Check sheet for the modelled part. Datum: model origin and axes. Units: mm. A direction names the side the tool comes from. Give positions to 0.01 mm unless a question says otherwise; leave off trailing zeros. Write each loop counter-clockwise with the first axis right and the second up, starting at its lowest first coordinate (ties: lowest second). Pieces come first, ordered by that corner, then holes. Notation, with made-up numbers: (75.5, 41.25) -> (112.5, 41.25) arc R20 ccw to (112.5, 77.25) -> close; hole circle Ø11 at (5, 80.25). An arc over 180 degrees is marked (long way). Use a Markdown table: item, result. Add a question column.
1. Gauge pin test, flat ends, axial feed: P1, Ø17.5, axis at x = -26.86, z = 15.88, coming from the -Y side; P2, Ø10, axis at x = -23, z = 25, coming from the +Y side; P3, Ø13.5, axis at y = -17.5, z = 11, coming from the -X side. Record the tip position at first contact, or that the pin passes through.
2. Scan lines: probe 1 along Y at (x, z) = (-24, 23); probe 2 along Y at (x, z) = (43.5, 29); probe 3 along X at (y, z) = (-3, 13). Record each from-to range of solid material in increasing order. Write a range as [from, to].
3. Cross-section at D-D (y = 13). Enter the section's corners in (x, z), then the cut area to 3 significant figures.
4. Cross-section at C-C (x = -23.5). Enter the section's corners in (y, z).
5. Set-up check for faces 1 (the flat face through (-22, 4.854, 19)), 2 (the flat face through (-22, -5.941, 19)), 3 (the flat face through (28, 0, 16)): record each of +Z, -Z, +X, -X, +Y, -Y from which the full face is reachable in a straight line by a thin tool's end or side.
6. Release check for a two-part mould opening along X. For faces 4 (the flat face through (-7, -23.086, 16)), 5 (the flat face through (0, 29, 16)), 6 (the cylindrical face through (-21.466, -0.619, 15.638)), 7 (the flat face through (-38.161, -1, 16)) record: released by +X, released by -X, zero draft, split by the parting line, or undercut.
7. Cross-section at A-A (z = 23). Enter the section's corners in (x, y) (3 decimals).
from build123d import *
from OCP.BRepFilletAPI import BRepFilletAPI_MakeChamfer

# Parameters (mm, degrees)
BOSS_EXTRUDE1_DEPTH          = 31.75
F_3_8_0_375_DIAMETER_HOLE1_D = 10.795
FILLET1_R                    = 1.27
FILLET2_R                    = 6.35
CHAMFER1_SIZE                = 0.254
CHAMFER1_SIZE2               = 0.321383695


with BuildPart() as part:
    # Sketch1 → Boss-Extrude1 (new body)
    with BuildSketch(Plane.XY):
        Polygon((0, 0), (50.8, 0), (50.8, -9.525), (-3.3628076, -23.086314), (-11.6178076, -23.086314), (-11.6178076, -5.941314), (-38.1608076, -5.941314), (-38.1608076, 4.853686), (-15.3008076, 4.853686), (-6.35, 50.8), (0, 50.8), align=None)
    extrude(amount=BOSS_EXTRUDE1_DEPTH)

    # 3/8 (0.375) Diameter Hole1 (through all)
    with Locations(Plane(origin=(0, 4.853686, 0), x_dir=(1, 0, 0), z_dir=(0, 1, 0))):
        with Locations((-26.8578076, -15.875)):
            Hole(F_3_8_0_375_DIAMETER_HOLE1_D / 2)

    # Fillet1
    fillet1_edges = [part.edges().sort_by_distance(p)[0] for p in [
        (-15.3008076, 4.853686, 15.875),
    ]]
    fillet(fillet1_edges, radius=FILLET1_R)

    # Fillet2
    fillet2_edges = [part.edges().sort_by_distance(p)[0] for p in [
        (0, 0, 15.875),
    ]]
    fillet(fillet2_edges, radius=FILLET2_R)

    # Chamfer1: one chamfer whose edges measure the first distance from different faces: ONE call of the kernel's chamfer builder (chamfer() names one face for all edges)
    chamfer1_edges_1 = [part.edges().sort_by_distance(p)[0] for p in [
        (28.575, 0, 0),
        (50.8, -4.7625, 0),
        (23.7185962, -16.305657, 0),
        (-7.4903076, -23.086314, 0),
        (-11.6178076, -14.513814, 0),
        (-10.725353572, 28.340421149, 31.75),
        (-24.8893076, -5.941314, 0),
        (-38.1608076, -0.543814, 0),
        (-10.725353572, 28.340421149, 0),
        (-3.175, 50.8, 0),
        (50.8, 0, 15.875),
        (-38.1608076, -5.941314, 15.875),
        (-38.1608076, 4.853686, 15.875),
        (0, 50.8, 15.875),
        (-38.1608076, -0.543814, 31.75),
        (-24.8893076, -5.941314, 31.75),
        (-11.6178076, -14.513814, 31.75),
        (-7.4903076, -23.086314, 31.75),
        (23.7185962, -16.305657, 31.75),
        (-27.254040401, 4.853686, 0),
        (-27.254040401, 4.853686, 31.75),
        (50.8, -4.7625, 31.75),
        (-15.539656801, 5.143555524, 0),
        (-15.539656801, 5.143555524, 31.75),
        (28.575, 0, 31.75),
        (0, 28.575, 0),
        (0, 28.575, 31.75),
        (1.859871939, 1.859871939, 0),
        (1.859871939, 1.859871939, 31.75),
        (-3.175, 50.8, 31.75),
    ]]
    chamfer1_edges_2 = [part.edges().sort_by_distance(p)[0] for p in [
        (-6.35, 50.8, 15.875),
    ]]
    chamfer1_side_2 = [part.faces().sort_by_distance(p)[0] for p in [
        (-3.175, 50.8, 15.875),
    ]]
    chamfer1 = BRepFilletAPI_MakeChamfer(part.part.solid().wrapped)
    for e in chamfer1_edges_1:
        chamfer1.Add(CHAMFER1_SIZE, e.wrapped)
    for e in chamfer1_edges_2:
        chamfer1.Add(CHAMFER1_SIZE, CHAMFER1_SIZE2, e.wrapped, chamfer1_side_2[0].wrapped)  # the first distance lies on this face
    add(Compound.cast(chamfer1.Shape()), mode=Mode.REPLACE)


solid = part.part
Worked answers:
| question | item | result |
|---|---|---|
| 1 | P1 | stops at y = -5.94 |
| 1 | P2 | stops at y = 4.85 |
| 1 | P3 | stops at x = -11.62 |
| 2 | probe 1 | y = [-5.94, 4.85] |
| 2 | probe 2 | y = [-11.35, 0] |
| 2 | probe 3 | x = [-38.16, -31.43], [-22.29, 50.8] |
| 3 | outline | (-13.71, 0.25) -> (-13.46, 0) -> (-0.25, 0) -> (0, 0.25) -> (0, 31.5) -> (-0.25, 31.75) -> (-13.46, 31.75) -> (-13.71, 31.5) -> close |
| 3 | area | 435 mm² |
| 4 | outline | (-5.94, 0.25) -> (-5.69, 0) -> (4.6, 0) -> (4.85, 0.25) -> (4.85, 11.65) -> (-5.94, 11.65) -> close; (-5.94, 20.1) -> (4.85, 20.1) -> (4.85, 31.5) -> (4.6, 31.75) -> (-5.69, 31.75) -> (-5.94, 31.5) -> close |
| 5 | face 1 | +Z, -Z, -X, +Y |
| 5 | face 2 | +Z, -Z, -X, -Y |
| 5 | face 3 | +Z, -Z, +X, +Y |
| 6 | face 4 | zero draft |
| 6 | face 5 | released by +X |
| 6 | face 6 | undercut |
| 6 | face 7 | released by -X |
| 7 | outline | (-38.161, -5.687) -> (-37.907, -5.941) -> (-11.618, -5.941) -> (-11.618, -23.086) -> (-3.363, -23.086) -> (50.8, -9.525) -> (50.8, -0.254) -> (50.546, 0) -> (6.35, 0) arc R6.35 cw to (0, 6.35) -> (0, 50.546) -> (-0.254, 50.8) -> (-6.096, 50.8) -> (-6.411, 50.485) -> (-15.101, 5.881) arc R1.27 cw to (-16.347, 4.854) -> (-37.907, 4.854) -> (-38.161, 4.6) -> close |
